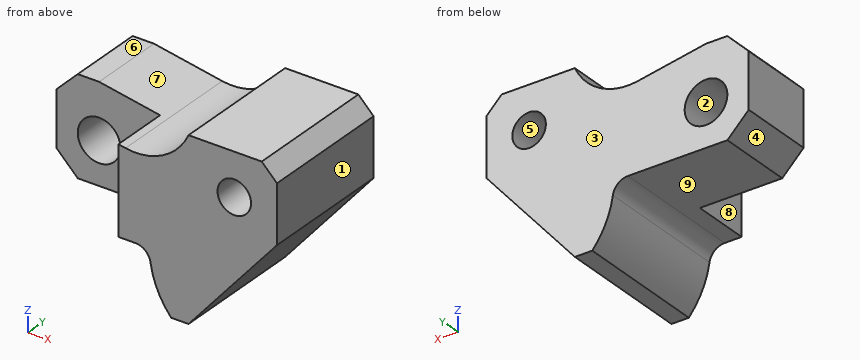
```python
from build123d import *

# Parameters (mm, degrees)
F0_R     = 7
F1_DEPTH = 44
F2_R     = 7
F3_DEPTH = 19
F2_R_2   = 5.5
F4_DEPTH = 44.001


with BuildPart() as f1:
    # F0 (on Front) → F1 (new body)
    with BuildSketch(Plane.XZ):
        with BuildLine():
            Line((-7, 18), (-14, 11))
            Line((-14, 11), (-14, -7))
            Line((-14, -7), (-7, -14))
            Line((-7, -14), (25.575539, -14))
            ThreePointArc((25.575539, -14), (28.840775, -15.213414), (30.521178, -18.264706))
            ThreePointArc((30.521178, -18.264706), (32.858008, -26.115672), (37.29698, -33))
            Line((37.29698, -33), (43, -33))
            Line((43, -33), (72, 1))
            Line((72, 1), (72, 20))
            Line((72, 20), (67, 25))
            Line((67, 25), (43, 25))
            ThreePointArc((43, 25), (34.561099, 15.982044), (22.361381, 14.057085))
            Line((22.361381, 14.057085), (0, 18))
            Line((0, 18), (-7, 18))
        make_face()
        Circle(F0_R, mode=Mode.SUBTRACT)
    extrude(amount=F1_DEPTH)

    # F2 (on face) → F3 (cut)
    with BuildSketch(Plane.XZ.offset(44)):
        Polygon((20, -14), (20, 14.47346), (0, 18), (-7, 18), (-14, 11), (-14, -7), (-7, -14), align=None)
        Circle(F2_R, mode=Mode.SUBTRACT)
    extrude(amount=-F3_DEPTH, mode=Mode.SUBTRACT)

    # F2 (on face) → F4 (cut, through all)
    with BuildSketch(Plane.XZ.offset(44)):
        with Locations((58, 11)):
            Circle(F2_R_2)
    extrude(amount=-F4_DEPTH, mode=Mode.SUBTRACT)


solid = f1.part
```
The listing builds one solid part. Answer for the finished solid, in the listing's coordinates (mm). Face numbers are marked on the shaded views. A direction names the side the tool comes from. Give positions to 0.01 mm unless a question says otherwise; leave off trailing zeros. Loops run counter-clockwise (first coordinate to the right, second up) from the corner with the lowest first, then second, coordinate; pieces in that order, holes last. Notation, with made-up numbers: M 42,1.25 L 87,1.25 A23 ccw 87,39.25 Z; hole C -18,77.25 d9. An arc over 180 degrees is marked long. One line per item, written item: value.
1. Find the intervals of material crossed by probe 1 along Z at (x, y) = (0, -13); probe 2 along Y at (x, z) = (9, -13); probe 3 along Z at (x, y) = (58, -20), in increasing order.
Found:
probe 1: -14 to -7, 7 to 18
probe 2: -25 to 0
probe 3: -15.41 to 5.5, 16.5 to 25
2. Section A-A on x = 3.5 is taken. Determine the outline of the cut face in (y, z).
Found:
outline: M -25,-14 L 0,-14 L 0,-6.06 L -25,-6.06 Z; M -25,6.06 L 0,6.06 L 0,17.38 L -25,17.38 Z
3. For the marked faces 5, 6, 7, 8 and 9, determine the directions among +Z, -Z, +X, -X, +Y, -Y from which every point of the face is accessible in a straight line to the end or side of a thin tool.
Found:
face 5: +Y, -Y
face 6: +Z, -X, +Y, -Y
face 7: +Z, +Y, -Y
face 8: +Z, -Z, -X, -Y
face 9: -Z, -X, +Y, -Y
4. Section D-D on y = -22 is taken. Determine the outline of the cut face in (x, z), plus the area to 3 significant figures.
Found:
outline: M -14,-7 L -7,-14 L 25.58,-14 A5 cw 30.52,-18.26 A29 ccw 37.3,-33 L 43,-33 L 72,1 L 72,20 L 67,25 L 43,25 A19 cw 22.36,14.06 L 0,18 L -7,18 L -14,11 Z; hole C 0,0 d14; hole C 58,11 d11
area: 2,830 mm^2
5. Section B-B on y = -39.5 is taken. Determine the outline of the cut face in (x, z), plus the area to 3 significant figures.
Found:
outline: M 20,-14 L 25.58,-14 A5 cw 30.52,-18.26 A29 ccw 37.3,-33 L 43,-33 L 72,1 L 72,20 L 67,25 L 43,25 A19 cw 22.36,14.06 L 20,14.47 Z; hole C 58,11 d11
area: 1,980 mm^2
6. Section C-C on z = 0 is taken. Determine the outline of the cut face in (x, y), plus the area to 3 significant figures.
Found:
outline: M -14,-25 L -7,-25 L -7,0 L -14,0 Z; M 7,-25 L 20,-25 L 20,-44 L 71.15,-44 L 71.15,0 L 7,0 Z
area: 2,750 mm^2
7. For a pull along X with two mould halves and no side action, classify the marked faces 1, 2, 3 and 4 as pulls with the +X half, pulls with the -X half, needs draft (parallel to the pull), parting line crosses it, or undercut.
Found:
face 1: pulls with the +X half
face 2: undercut
face 3: needs draft
face 4: pulls with the -X half
8. Each of these flat-tipped pins is pushed along its axis until it touches: P1, Ø4, axis at y = -16.5, z = -16.5, coming from the -X side (3 decimals); P2, Ø16, axis at x = 2.5, z = 9, coming from the -Y side; P3, Ø2, axis at y = -27.5, z = 18, coming from the -X side. Where does it stop, or does it pass through?
Found:
P1: x = 27.755
P2: y = -25
P3: x = 36.26
